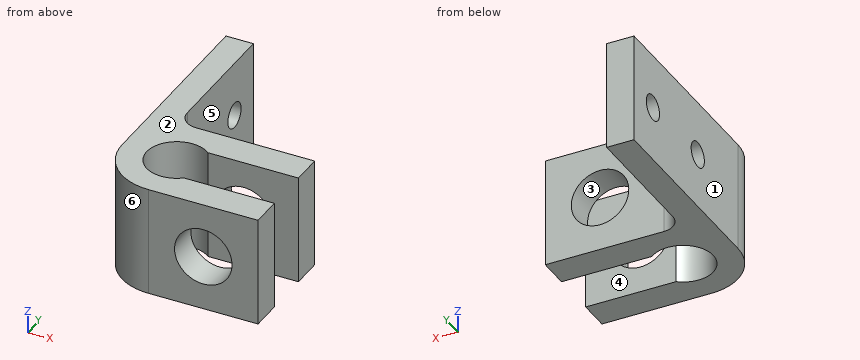
```python
from build123d import *

# Parameters (mm, degrees)
BOSS_EXTRUDE1_DEPTH     = 12
CUT_EXTRUDE1_DEPTH      = 28.784887979
CUT_EXTRUDE1_DEPTH_BACK = 28.784887979
SKETCH2_R               = 3.15
CUT_EXTRUDE2_REACH      = 32.854
SKETCH3_R               = 1.4


with BuildPart() as part:
    # Sketch1 → Boss-Extrude1 (new body)
    with BuildSketch(Plane.XY):
        with BuildLine():
            Line((-1, 6), (12, 6))
            Line((12, 6), (12, 2.552710574))
            Line((12, 2.552710574), (2.091331807, 2.552710574))
            ThreePointArc((2.091331807, 2.552710574), (-3.3, 0), (2.091331807, -2.552710574))
            Line((2.091331807, -2.552710574), (12, -2.552710574))
            Line((12, -2.552710574), (12, -6))
            Line((12, -6), (0, -6))
            ThreePointArc((0, -6), (-4.242640687, -4.242640687), (-6, 0))
            Line((-6, 0), (-6, 22))
            Line((-6, 22), (-3, 22))
            Line((-3, 22), (-3, 8))
            ThreePointArc((-3, 8), (-2.414213562, 6.585786438), (-1, 6))
        make_face()
    extrude(amount=BOSS_EXTRUDE1_DEPTH)

    # Sketch2 → Cut-Extrude1 (cut, two sides: drawn at the far end of the back side and taken through both)
    with BuildSketch(Plane(origin=(0, 0, 0), x_dir=(1, 0, 0), z_dir=(0, 1, 0)).offset(-CUT_EXTRUDE1_DEPTH_BACK)):
        with Locations(Location((6, -6, 0), (0, 0, 270))):
            Circle(SKETCH2_R)
    extrude(amount=CUT_EXTRUDE1_DEPTH + CUT_EXTRUDE1_DEPTH_BACK, mode=Mode.SUBTRACT)

    # Sketch3 → Cut-Extrude2 (cut, up to next)
    with BuildSketch(Plane.ZY.offset(6), mode=Mode.PRIVATE) as cut_extrude2_sk1:
        with Locations((6, 18)):
            Circle(SKETCH3_R)
    cut_extrude2_tool1 = extrude(cut_extrude2_sk1.sketch, amount=-CUT_EXTRUDE2_REACH, mode=Mode.PRIVATE) & part.part
    # Sketch3 → Cut-Extrude2 (cut, up to next)
    with BuildSketch(Plane.ZY.offset(6), mode=Mode.PRIVATE) as cut_extrude2_sk2:
        with Locations((6, 8.5)):
            Circle(SKETCH3_R)
    cut_extrude2_tool2 = extrude(cut_extrude2_sk2.sketch, amount=-CUT_EXTRUDE2_REACH, mode=Mode.PRIVATE) & part.part
    add(cut_extrude2_tool1.solids().sort_by_distance((-6, 18, 6))[0], mode=Mode.SUBTRACT)
    add(cut_extrude2_tool2.solids().sort_by_distance((-6, 8.5, 6))[0], mode=Mode.SUBTRACT)


solid = part.part
```
Read the model definition and answer for the solid it produces. Units are mm, in the model's axes. Face numbers are marked on the shaded views. A direction names the side the tool comes from. Give positions to 0.01 mm unless a question says otherwise; leave off trailing zeros. Order: outer loops, then holes, each group sorted by start corner. A loop starts at its lowest first (then second) coordinate and runs counter-clockwise, first axis right, second up.
(1) Straight lines are drawn through the part: L1, parallel to X at y = 4.3, z = 6; L2, parallel to Y at x = 0, z = 8.25; L3, parallel to Y at x = -4.2, z = 6. For each, find the intervals that lie inside material, in ascending order.
(2) Find section C-C (z = 6). Give the vertices of the cut face in (x, y).
(3) Find section D-D (x = 2.5). Give the vertices of the cut face in (y, z).
(4) Given pin 1 (5 mm diameter, centred on x = 7, z = 8, fed in from +Y); pin 2 (2.5 mm diameter, centred on y = 18, z = 6, fed in from +X); pin 3 (3 mm diameter, centred on y = 0, z = 2.5, fed in from +X), each flat-ended and moving along its own axis, determine where each tip first touches the part or whether it passes through.
(5) For the marked faces 4, 5 and 6, determine the directions among +Z, -Z, +X, -X, +Y, -Y from which every point of the face is accessible in a straight line to the end or side of a thin tool.
(6) For a pull along X with two mould halves and no side action, classify the marked faces 1, 2 and 3 as released by +X, released by -X, zero draft, split by the parting line, or undercut.
(7) Find section B-B (x = 6). Give the vertices of the cut face in (y, z), plus the area to 3 significant figures.
(8) Find section A-A (y = 8.5). Give the vertices of the cut face in (x, z), plus the area to 3 significant figures.
Result sheet:
1. L1: x = -6 to 2.85, 9.15 to 12
1. L2: y = -6 to -3.3, 3.3 to 6
1. L3: y = -4.28 to 7.1, 9.9 to 16.6, 19.4 to 22
2. outline: (-6, 0) arc R6 ccw to (0, -6) - (2.85, -6) - (2.85, -2.55) - (2.09, -2.55) arc R3.3 cw (long way) to (2.09, 2.55) - (2.85, 2.55) - (2.85, 6) - (-1, 6) arc R2 cw to (-2.79, 7.1) - (-6, 7.1) - close; (-6, 9.9) - (-3, 9.9) - (-3, 16.6) - (-6, 16.6) - close; (-6, 19.4) - (-3, 19.4) - (-3, 22) - (-6, 22) - close; (9.15, -6) - (12, -6) - (12, -2.55) - (9.15, -2.55) - close; (9.15, 2.55) - (12, 2.55) - (12, 6) - (9.15, 6) - close
3. outline: (-6, 0) - (-2.55, 0) - (-2.55, 12) - (-6, 12) - close; (2.55, 0) - (6, 0) - (6, 12) - (2.55, 12) - close
4. pin 1: stops at y = 6
4. pin 2: passes through
4. pin 3: stops at x = -2.94
5. face 4: +Z, -Z, +X
5. face 5: +Z, -Z, +X, +Y
5. face 6: +Z, -Z, -X, -Y
6. face 1: released by -X
6. face 2: zero draft
6. face 3: undercut
7. outline: (-6, 0) - (-2.55, 0) - (-2.55, 2.85) - (-6, 2.85) - close; (-6, 9.15) - (-2.55, 9.15) - (-2.55, 12) - (-6, 12) - close; (2.55, 0) - (6, 0) - (6, 2.85) - (2.55, 2.85) - close; (2.55, 9.15) - (6, 9.15) - (6, 12) - (2.55, 12) - close
7. area: 39.3 mm2
8. outline: (-6, 0) - (-3, 0) - (-3, 4.6) - (-6, 4.6) - close; (-6, 7.4) - (-3, 7.4) - (-3, 12) - (-6, 12) - close
8. area: 27.6 mm2
